For this review, take the finished solid that the model builds, in its own axes (mm). Face numbers are marked on the shaded views. A direction names the side the tool comes from. Round coordinates to 2 decimals unless told otherwise and drop trailing zeros. Write each loop counter-clockwise with the first axis right and the second up, starting at its lowest first coordinate (ties: lowest second). Pieces come first, ordered by that corner, then holes.
from build123d import *

# Parameters (mm, degrees)
F0_R     = 37.5
F0_R_2   = 25
F1_DEPTH = 35
F2_W     = 20
F2_H     = 35
F3_DEPTH = 69
F4_SIZE  = 9.99999


# Not quite as in the source:
# - a fillet or chamfer is up to 0.001 mm smaller than in the source, because OpenCascade refuses the exact size


with BuildPart() as f1:
    # F0 (on Top) → F1 (new body)
    with BuildSketch(Plane.XY):
        Circle(F0_R)
        Circle(F0_R_2, mode=Mode.SUBTRACT)
    extrude(amount=F1_DEPTH)

    # F2 (on Front) → F3 (join)
    with BuildSketch(Plane.XZ):
        with Locations((0, 17.5)):
            Rectangle(F2_W, F2_H)
    extrude(amount=F3_DEPTH)

    # F4 (size 10 in the source; OpenCascade refuses exactly that, so slightly less here)
    f4_edges = [f1.edges().sort_by_distance(p)[0] for p in [
        (-10, -69, 17.5),
        (10, -69, 17.5),
    ]]
    chamfer(f4_edges, length=F4_SIZE)


solid = f1.part
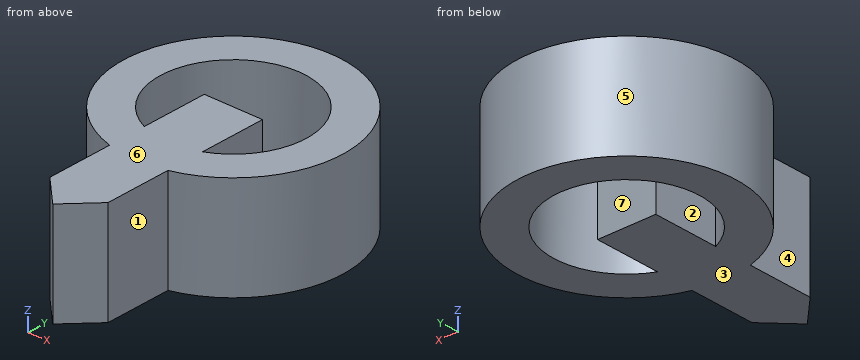
(1) We need section D-D, the plane y = -21.5. Give the boundary of the cut face in (x, z), and give its area (3 significant figures).
Geometry check:
outline: (-30.72, 0) - (-12.76, 0) - (-12.76, 35) - (-30.72, 35) - close; (-10, 0) - (10, 0) - (10, 35) - (-10, 35) - close; (12.76, 0) - (30.72, 0) - (30.72, 35) - (12.76, 35) - close
area: 1,960 mm2
(2) For the marked faces 1, 2, 3 and 4, list the 3-axis set-ups (+Z, -Z, +X, -X, +Y, -Y) from which the entire face can be reached by the end or side of a thin tool; tool diameter is ignored.
Geometry check:
face 1: +Z, -Z, +X, -Y
face 2: +Z, -Z
face 3: -Z, +X, -X, +Y, -Y
face 4: +Z, -Z, -X, -Y
(3) For pin 1 Ø3 at (x, z) = (21, 29.5) entering from -Y; pin 2 Ø6 at (x, z) = (-28, 6.5) entering from -Y; pin 3 Ø4 at (y, z) = (19.5, 10.5) entering from -X; pin 4 Ø1 at (x, y) = (-24, -31) entering from +Z, all flat-tipped, find the tip position at first contact; note any pin that passes through.
Geometry check:
pin 1: stops at y = -32.03
pin 2: stops at y = -27.95
pin 3: stops at x = -33.17
pin 4: passes through
(4) We need section B-B, the plane x = 20. Give the boundary of the cut face in (y, z).
Geometry check:
outline: (-31.72, 0) - (-15, 0) - (-15, 35) - (-31.72, 35) - close; (15, 0) - (31.72, 0) - (31.72, 35) - (15, 35) - close
(5) For line 1 along X through (y, z) = (-16, 18); line 2 along X through (y, z) = (-2, 7); line 3 along X through (y, z) = (-39, 26.5), list the stretches that pass through material, from the lowest coordinate up.
Geometry check:
line 1: x = -33.92 to -19.21, -10 to 10, 19.21 to 33.92
line 2: x = -37.45 to -24.92, -10 to 10, 24.92 to 37.45
line 3: x = -10 to 10
(6) Mouldability with a two-part tool opening along Y and no side actions: class the marked faces 5, 6 and 7 as pulls with the +Y half, pulls with the -Y half, needs draft (parallel to the pull), parting line crosses it, or undercut.
Geometry check:
face 5: parting line crosses it
face 6: needs draft
face 7: undercut
(7) We need section C-C, the plane y = 19. Give the boundary of the cut face in (x, z), and give its area (3 significant figures).
Geometry check:
outline: (-32.33, 0) - (-16.25, 0) - (-16.25, 35) - (-32.33, 35) - close; (16.25, 0) - (32.33, 0) - (32.33, 35) - (16.25, 35) - close
area: 1,130 mm2
